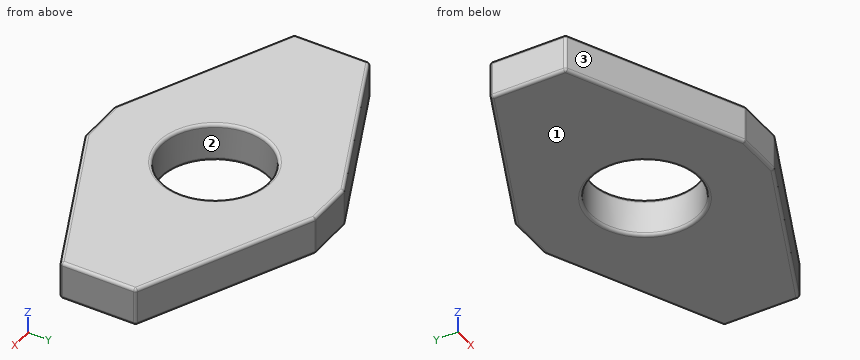
from build123d import *

# Parameters (mm, degrees)
F0_R     = 8.89
F1_DEPTH = 6.35
F2_R     = 0.508


with BuildPart() as f1:
    # F0 (on Top) → F1 (new body)
    with BuildSketch(Plane.XY):
        Polygon((0, -12.812661), (-27.827339, 0), (-35.672661, 0), (-63.5, -12.812661), (-63.5, -25.287339), (-35.672661, -38.1), (-27.827339, -38.1), (0, -25.287339), align=None)
        with Locations((-31.75, -19.05)):
            Circle(F0_R, mode=Mode.SUBTRACT)
    extrude(amount=F1_DEPTH)

    # F2
    f2_edges = [f1.edges().sort_by_distance(p)[0] for p in [
        (-63.5, -25.287339, 3.175),
        (-35.672661, -38.1, 3.175),
        (-49.58633, -31.693669, 0),
        (-49.58633, -31.693669, 6.35),
        (-13.91367, -6.406331, 6.35),
        (-31.75, 0, 6.35),
        (-49.58633, -6.406331, 6.35),
        (-63.5, -19.05, 6.35),
        (-31.75, -38.1, 6.35),
        (-13.91367, -31.693669, 6.35),
        (0, -19.05, 6.35),
        (-40.64, -19.05, 6.35),
        (-13.91367, -6.406331, 0),
        (-31.75, 0, 0),
        (-49.58633, -6.406331, 0),
        (-63.5, -19.05, 0),
        (-31.75, -38.1, 0),
        (-13.91367, -31.693669, 0),
        (0, -19.05, 0),
        (-40.64, -19.05, 0),
        (-63.5, -12.812661, 3.175),
        (-35.672661, 0, 3.175),
        (-27.827339, 0, 3.175),
        (0, -12.812661, 3.175),
        (0, -25.287339, 3.175),
        (-27.827339, -38.1, 3.175),
    ]]
    fillet(f2_edges, radius=F2_R)


solid = f1.part
Read the model definition and answer for the solid it produces. Units are mm, in the model's axes. Face numbers are marked on the shaded views. Coordinates: 2 decimals unless noted, no trailing zeros. Write each loop counter-clockwise with the first axis right and the second up, starting at its lowest first coordinate (ties: lowest second). Pieces come first, ordered by that corner, then holes. Notation, with made-up numbers: (75, -7.5) -> (128, -7.5) arc R11 cw to (128, 12.5) -> close; hole circle Ø10 at (-13, 77). An arc over 180 degrees is marked (long way). Return JSON: item names as keys, results as strings.
(1) This flat-tipped pin is pushed along its axis until it touches: P1, Ø1, axis at x = -38.5, z = 1.5, coming from the -Y side. Where does it stop, or does it pass through?
Answers below:
{"P1": "y = -37.03"}
(2) Consider line 1 along Y through (x, z) = (-31.75, 2.7); line 2 along X through (y, z) = (-13, 2.75); line 3 along Y through (x, z) = (-25, 1). Determine where each line is inside the solid, lowest interval first. Write a range as from..to.
Answers below:
{"line 1": "-38.1..-27.94, -10.16..0", "line 2": "-63.48..-38.26, -25.24..-0.02", "line 3": "-36.8..-24.84, -13.26..-1.3"}
(3) The part is cut by section B-B on x = -31.75. Give the vertices of the cut face in (y, z).
Answers below:
{"outline": "(-38.1, 0.51) arc R0.51 ccw to (-37.59, 0) -> (-28.45, 0) arc R0.51 ccw to (-27.94, 0.51) -> (-27.94, 5.84) arc R0.51 ccw to (-28.45, 6.35) -> (-37.59, 6.35) arc R0.51 ccw to (-38.1, 5.84) -> close; (-10.16, 0.51) arc R0.51 ccw to (-9.65, 0) -> (-0.51, 0) arc R0.51 ccw to (0, 0.51) -> (0, 5.84) arc R0.51 ccw to (-0.51, 6.35) -> (-9.65, 6.35) arc R0.51 ccw to (-10.16, 5.84) -> close"}
(4) The part is cut by section C-C on z = 3.75. Give the vertices of the cut face in (x, y).
Answers below:
{"outline": "(-63.5, -24.96) arc R0.51 ccw to (-63.2, -25.42) -> (-35.77, -38.05) arc R0.51 ccw to (-35.56, -38.1) -> (-27.94, -38.1) arc R0.51 ccw to (-27.73, -38.05) -> (-0.3, -25.42) arc R0.51 ccw to (0, -24.96) -> (0, -13.14) arc R0.51 ccw to (-0.3, -12.68) -> (-27.73, -0.05) arc R0.51 ccw to (-27.94, 0) -> (-35.56, 0) arc R0.51 ccw to (-35.77, -0.05) -> (-63.2, -12.68) arc R0.51 ccw to (-63.5, -13.14) -> close; hole circle Ø17.78 at (-31.75, -19.05)"}
(5) The part is cut by section A-A on y = -19.05. Give the vertices of the cut face in (x, z), then the cut area to 3 significant figures.
Answers below:
{"outline": "(-63.5, 0.51) arc R0.51 ccw to (-62.99, 0) -> (-41.15, 0) arc R0.51 ccw to (-40.64, 0.51) -> (-40.64, 5.84) arc R0.51 ccw to (-41.15, 6.35) -> (-62.99, 6.35) arc R0.51 ccw to (-63.5, 5.84) -> close; (-22.86, 0.51) arc R0.51 ccw to (-22.35, 0) -> (-0.51, 0) arc R0.51 ccw to (0, 0.51) -> (0, 5.84) arc R0.51 ccw to (-0.51, 6.35) -> (-22.35, 6.35) arc R0.51 ccw to (-22.86, 5.84) -> close", "area": "290 mm^2"}
(6) For a pull along X with two mould halves and no side action, classify the marked faces 1, 2 and 3 as pulls with the +X half, pulls with the -X half, needs draft (parallel to the pull), parting line crosses it, or undercut.
Answers below:
{"face 1": "needs draft", "face 2": "undercut", "face 3": "pulls with the -X half"}
